Can you work these out from the model? Positions are in its coordinate system, mm. A direction names the side the tool comes from. Coordinates: 2 decimals unless noted, no trailing zeros. Order: outer loops, then holes, each group sorted by start corner. A loop starts at its lowest first (then second) coordinate and runs counter-clockwise, first axis right, second up. Notation, with made-up numbers: (29, -28.75) - (60, -28.75) arc R22 cw to (60, -0.75) - close; hole circle Ø4 at (0.5, 53). An arc over 180 degrees is marked (long way). Return JSON: item names as keys, results as strings. Group by question number.
1) Imagine slicing it at B-B (z = 17.5). Write out the boundary of the cut face in (x, y), and give its area (3 significant figures).
2) Imagine slicing it at A-A (x = -27). Write out the boundary of the cut face in (y, z), and give its area (3 significant figures).
3) Imagine slicing it at C-C (y = 25). Write out the boundary of the cut face in (x, z).
4) If I drill on line 1 along Y through (x, z) = (42.5, 7.5); line 2 along Y through (x, z) = (14.5, 8.25); line 3 along X through (y, z) = (-37, 5.5), over which ranges is the centre line in solid material (lowest first)?
5) If we mould it in two halves opening along X, with no side actions, what happens to faces 4 (the face through (-1, 1, 0)), 5 (the face through (-52.036, 0.007, 17.621)), 6 (the face through (-41.39, 25.46, 5.99))? For each: pulls with the +X half, pulls with the -X half, needs draft (parallel to the pull), parting line crosses it, or undercut.
6) Which directions (+Z, -Z, +X, -X, +Y, -Y) give clear straight access to the entire face, cutting with the end or side of a thin tool? Please do faces 1 (the face through (53.5, 23, 4)), 2 (the face through (-49.65, 0, 9)), 3 (the face through (-49.5, 17, 1)).
7) For pin 1 Ø6 at (x, z) = (-41.5, 15) entering from +Y; pin 2 Ø1.9 at (x, y) = (42, 25) entering from +Z; pin 3 Ø6 at (x, y) = (6, 12) entering from +Z; pin 4 Ø3.5 at (x, z) = (52, 13) entering from -Y, each with a flat end and sliding along its axis, tell me the tip position at first contact or that it passes through.
Solid Edge part; units mm, degrees
sketch "Sketch1" plane through (0, 0, 0) normal (0, 0, 1) x (1, 0, 0)
  line L0 (19.5, 20) -> (19.5, 15)
  line L1 (19.5, 15) -> (49.5, 15)
  line L2 (49.5, 15) -> (49.5, 20)
  line L3 (49.5, 20) -> (19.5, 20)
  line L4 (-7, -39.85) -> (-5, -39.85)
  line L5 (-5, -39.85) -> (-5, -14.85)
  line L6 (-5, -14.85) -> (-7, -14.85)
  line L7 (-7, -14.85) -> (-7, -39.85)
  line L8 (53.5, 43.85) -> (-53.5, 43.85)
  line L9 (-53.5, 43.85) -> (-53.5, -43.85)
  line L10 (-53.5, -43.85) -> (53.5, -43.85)
  line L11 (53.5, -43.85) -> (53.5, 43.85)
  line L12 (7, -39.85) -> (5, -39.85)
  line L13 (5, -39.85) -> (5, -14.85)
  line L14 (5, -14.85) -> (7, -14.85)
  line L15 (7, -14.85) -> (7, -39.85)
  line L16 (-49.5, 20) -> (-19.5, 20)
  line L17 (-19.5, 20) -> (-19.5, 15)
  line L18 (-19.5, 15) -> (-49.5, 15)
  line L19 (-49.5, 15) -> (-49.5, 20)
extrude "ExtrudedProtrusion_2" add sketch "Sketch1" along normal blind 10
sketch "Sketch2" plane through (0, 0, 10) normal (0, 0, 1) x (0, 1, 0)
  line L0 (41.5, -51.1) -> (-41.5, -51.1)
  line L1 (-41.5, -51.1) -> (-41.5, 51.1)
  line L2 (-41.5, 51.1) -> (41.5, 51.1)
  line L3 (41.5, 51.1) -> (41.5, -51.1)
  line L4 (-39.85, -7) -> (-39.85, -5)
  line L5 (-39.85, -5) -> (-14.85, -5)
  line L6 (-14.85, -5) -> (-14.85, -7)
  line L7 (-14.85, -7) -> (-39.85, -7)
  line L8 (15, 49.5) -> (20, 49.5)
  line L9 (20, 49.5) -> (20, 19.5)
  line L10 (20, 19.5) -> (15, 19.5)
  line L11 (15, 19.5) -> (15, 49.5)
  line L12 (-14.85, 5) -> (-14.85, 7)
  line L13 (-14.85, 7) -> (-39.85, 7)
  line L14 (-39.85, 7) -> (-39.85, 5)
  line L15 (-39.85, 5) -> (-14.85, 5)
  line L16 (15, -49.5) -> (20, -49.5)
  line L17 (20, -49.5) -> (20, -19.5)
  line L18 (20, -19.5) -> (15, -19.5)
  line L19 (15, -19.5) -> (15, -49.5)
extrude "ExtrudedCutout_1" cut sketch "Sketch2" against normal blind 7.9
sketch "Sketch3" plane through (0, 0, 10) normal (0, 0, 1) x (1, 0, 0)
  line L0 (-52.1, 42.45) -> (-52.1, -42.45)
  line L1 (-52.1, -42.45) -> (52.1, -42.45)
  line L2 (52.1, -42.45) -> (52.1, 42.45)
  line L3 (52.1, 42.45) -> (-52.1, 42.45)
  line L4 (53.5, 43.85) -> (-53.5, 43.85)
  line L5 (-53.5, 43.85) -> (-53.5, -43.85)
  line L6 (-53.5, -43.85) -> (53.5, -43.85)
  line L7 (53.5, -43.85) -> (53.5, 43.85)
extrude "ExtrudedCutout_2" cut sketch "Sketch3" against normal blind 1
sketch "Sketch4" plane through (0, 0, 2.1) normal (0, 0, 1) x (1, 0, 0)
  line L0 (-49.65, -5.6) -> (-49.65, 5.6)
  line L1 (-49.65, 5.6) -> (-51.1, 5.6)
  line L2 (-51.1, 5.6) -> (-51.1, -5.6)
  line L3 (-51.1, -5.6) -> (-49.65, -5.6)
extrude "ExtrudedProtrusion_3" add sketch "Sketch4" along normal blind 5
mirror "Mirror1" about plane through (0, 0, 0) normal (1, 0, 0) of "ExtrudedProtrusion_3"
sketch "Sketch5" plane through (-50.375, 0, 7.1) normal (0, 0, 1) x (0, 1, 0)
  line L0 (-2.4577, -0.725) -> (2.5423, -0.725)
  line L1 (2.5423, -0.725) -> (2.5423, 0.725)
  line L2 (2.5423, 0.725) -> (-2.4577, 0.725)
  line L3 (-2.4577, 0.725) -> (-2.4577, -0.725)
extrude "ExtrudedProtrusion_4" add sketch "Sketch5" along normal blind 8
mirror "Mirror2" about plane through (0, 0, 0) normal (1, 0, 0) of "ExtrudedProtrusion_4"
sketch "Sketch6" plane through (-50.375, -2.4577, 11.1) normal (0, -1, 0) x (0, 0, 1)
  line L0 (4, 2.675) -> (4, -0.725)
  line L1 (4, -0.725) -> (8, -0.725)
  line L2 (8, -0.725) -> (8, 0.675)
  line L3 (8, 0.675) -> (5, 2.675)
  line L4 (5, 2.675) -> (4, 2.675)
extrude "ExtrudedProtrusion_5" add sketch "Sketch6" against normal blind 5
mirror "Mirror3" about plane through (0, 0, 0) normal (1, 0, 0) of "ExtrudedProtrusion_5"
sketch "Sketch7" plane through (0, 0, 0) normal (0, 0, -1) x (0, 1, 0)
  line L0 (-4, 51.1) -> (4, 51.1)
  line L1 (4, 51.1) -> (4, 53.5)
  line L2 (4, 53.5) -> (-4, 53.5)
  line L3 (-4, 53.5) -> (-4, 51.1)
extrude "ExtrudedCutout_4" cut sketch "Sketch7" against normal blind 10
mirror "Mirror4" about plane through (0, 0, 0) normal (1, 0, 0) of "ExtrudedCutout_4"
sketch "Sketch8" plane through (0, 0, 2.1) normal (0, 0, 1) x (1, 0, 0)
  circle A0 centre (42.5, -25) radius 1.2
  circle A1 centre (42.5, -25) radius 2.4
  circle A2 centre (-42.5, -25) radius 2.4
  circle A3 centre (-42.5, -25) radius 1.2
  circle A4 centre (-42.5, 25) radius 1.2
  circle A5 centre (-42.5, 25) radius 2.4
  circle A6 centre (42.5, 25) radius 2.4
  circle A7 centre (42.5, 25) radius 1.2
extrude "ExtrudedProtrusion_6" add sketch "Sketch8" along normal blind 7.9
fillet "Round_1" radius 2 4 edges at (53.5, -43.85, 4.5) (53.5, 43.85, 4.5) (-53.5, 43.85, 4.5) (-53.5, -43.85, 4.5)
Calculated:
{
 "1": {"outline": "(-52.12, -2.46) - (-49.65, -2.46) - (-49.65, 2.54) - (-52.12, 2.54) - close; (49.65, -2.46) - (52.12, -2.46) - (52.12, 2.54) - (49.65, 2.54) - close", "area": "24.7 mm2"},
 "2": {"outline": "(-43.85, 0) - (15, 0) - (15, 2.1) - (-41.5, 2.1) - (-41.5, 10) - (-42.45, 10) - (-42.45, 9) - (-43.85, 9) - close; (20, 0) - (43.85, 0) - (43.85, 9) - (42.45, 9) - (42.45, 10) - (41.5, 10) - (41.5, 2.1) - (20, 2.1) - close", "area": "208 mm2"},
 "3": {"outline": "(-53.5, 0) - (53.5, 0) - (53.5, 9) - (52.1, 9) - (52.1, 10) - (51.1, 10) - (51.1, 2.1) - (44.9, 2.1) - (44.9, 10) - (43.7, 10) - (43.7, 2.1) - (41.3, 2.1) - (41.3, 10) - (40.1, 10) - (40.1, 2.1) - (-40.1, 2.1) - (-40.1, 10) - (-41.3, 10) - (-41.3, 2.1) - (-43.7, 2.1) - (-43.7, 10) - (-44.9, 10) - (-44.9, 2.1) - (-51.1, 2.1) - (-51.1, 10) - (-52.1, 10) - (-52.1, 9) - (-53.5, 9) - close"},
 "4": {"line 1": "-43.85 to -41.5, -27.4 to -26.2, -23.8 to -22.6, 22.6 to 23.8, 26.2 to 27.4, 41.5 to 43.85", "line 2": "-43.85 to -41.5, 41.5 to 43.85", "line 3": "-53.5 to -51.1, 51.1 to 53.5"},
 "5": {"face 4": "needs draft", "face 5": "pulls with the -X half", "face 6": "undercut"},
 "6": {"face 1": "+Z, -Z, +X, +Y, -Y", "face 2": "+Z", "face 3": "+Z, -Z"},
 "7": {"pin 1": "through", "pin 2": "z = 10", "pin 3": "z = 2.1", "pin 4": "y = -2.46"}
}
